Source: CAD feature listing. Evaluate the final solid. Frame: model axes, mm. Face numbers are marked on the shaded views. A direction names the side the tool comes from. Coordinates: 2 decimals unless noted, no trailing zeros. Loops run counter-clockwise (first coordinate to the right, second up) from the corner with the lowest first, then second, coordinate; pieces in that order, holes last. Notation, with made-up numbers: (69, 56.25) - (80, 56.25) arc R18 ccw to (80, 89.25) - close; hole circle Ø5 at (-32, 27.5). An arc over 180 degrees is marked (long way). Write item = value, one per line. Start each with the question number.
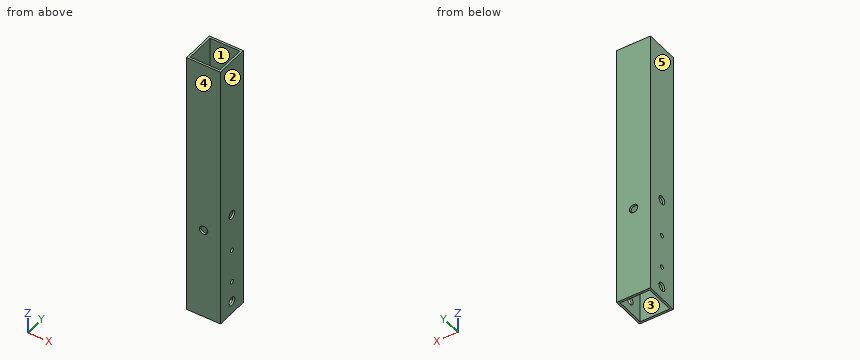
Autodesk Inventor part; units mm, degrees
ref_plane "YZ Plane" through (0, 0, 0) normal (1, 0, 0) x (0, 1, 0)
ref_plane "XZ Plane" through (0, 0, 0) normal (0, 1, 0) x (-1, 0, 0)
ref_plane "XY Plane" through (0, 0, 0) normal (0, 0, 1) x (1, 0, 0)
sketch "Sketch1" plane through (0, 0, 0) normal (0, 0, 1) x (1, 0, 0)
  line L0 (0, 0) -> (-11.1125, 0) construction
  line L1 (0, 0) -> (0, 11.1125) construction
  line L2 (-11.1125, 11.1125) -> (11.1125, 11.1125)
  line L3 (11.1125, 11.1125) -> (11.1125, -11.1125)
  line L4 (11.1125, -11.1125) -> (-11.1125, -11.1125)
  line L5 (-11.1125, -11.1125) -> (-11.1125, 11.1125)
  line L6 (-12.7, 12.7) -> (12.7, 12.7)
  line L7 (12.7, 12.7) -> (12.7, -12.7)
  line L8 (12.7, -12.7) -> (-12.7, -12.7)
  line L9 (-12.7, -12.7) -> (-12.7, 12.7)
  line L10 (-11.1125, 0) -> (-12.7, 0) construction
  line L11 (0, 11.1125) -> (0, 12.7) construction
  dimension "d0" = 25.4
  dimension "d1" = 1.5875
extrude "Extrusion1" add sketch "Sketch1" along normal blind 203.2
sketch "Sketch2" plane through (-12.7, 12.7, 0) normal (0, 1, 0) x (1, 0, 0)
  line L0 (12.7, 0) -> (12.7, -203.2) construction
  line L1 (25.4, 0) -> (25.4, -203.2) construction
  circle A0 centre (12.7, -69.85) radius 3.175
  dimension "d4" = 6.35
  dimension "d5" = 69.85
extrude "Extrusion2" cut sketch "Sketch2" against normal through all
sketch "Sketch3" plane through (12.7, -12.7, 0) normal (1, 0, 0) x (0, 0, -1)
  line L0 (0, 12.7) -> (-203.2, 12.7) construction
  line L1 (0, 23.8125) -> (-203.2, 23.8125) construction
  circle A0 centre (-79.375, 12.7) radius 3.175
  circle A1 centre (-9.525, 12.7) radius 3.175
  line L2 (0, 25.4) -> (0, 0)
  line L3 (-38.1, 23.8125) -> (-38.1, 12.7) construction
  circle A2 centre (-50.8, 12.7) radius 1.5875
  circle A3 centre (-25.4, 12.7) radius 1.5875
  dimension "d8" = 6.35
  dimension "d9" = 79.375
  dimension "d12" = 6.35
  dimension "d13" = 9.525
  dimension "d22" = 3.175
  dimension "d23" = 25.4
  dimension "d24" = 38.1
extrude "Extrusion3" cut sketch "Sketch3" against normal through all
properties part number "Upright" material "Aluminum 6061"
Item 1: Cut plane C-C (y = 8.5). Return the cut outline in (x, z), then the cut area to 3 significant figures.
Item 2: Reachability of the marked faces 1 and 2 from +Z, -Z, +X, -X, +Y, -Y: full face, straight path, thin tool, end or side. Return the list, or none.
Item 3: Cut plane A-A (x = 0). Return the cut outline in (y, z) (1 decimal).
Item 4: Cut plane B-B (z = 111). Return the cut outline in (x, y).
Item 5: Draft query along X for the marked faces 3, 4 and 5. Return one class per face: released by +X, released by -X, zero draft, split by the parting line, or undercut.
Item 6: Material intervals for L1, parallel to X at y = 11.55, z = 69.85 (3 decimals); L2, parallel to X at y = -4, z = 95, sorted ascending. Write a range as [from, to].
Responses:
q1.outline = (-12.7, 0) - (-11.11, 0) - (-11.11, 203.2) - (-12.7, 203.2) - close; (11.11, 0) - (12.7, 0) - (12.7, 203.2) - (11.11, 203.2) - close
q1.area = 645 mm2
q2.face_1 = +Z, -Z
q2.face_2 = +Z, -Z, +X, +Y, -Y
q3.outline = (-12.7, 0) - (-11.1, 0) - (-11.1, 66.7) - (-12.7, 66.7) - close; (-12.7, 73) - (-11.1, 73) - (-11.1, 203.2) - (-12.7, 203.2) - close; (11.1, 0) - (12.7, 0) - (12.7, 66.7) - (11.1, 66.7) - close; (11.1, 73) - (12.7, 73) - (12.7, 203.2) - (11.1, 203.2) - close
q4.outline = (-12.7, -12.7) - (12.7, -12.7) - (12.7, 12.7) - (-12.7, 12.7) - close; hole (-11.11, -11.11) - (11.11, -11.11) - (11.11, 11.11) - (-11.11, 11.11) - close
q5.face_3 = undercut
q5.face_4 = zero draft
q5.face_5 = released by -X
q6.L1 = [-12.7, -3.175], [3.175, 12.7]
q6.L2 = [-12.7, -11.11], [11.11, 12.7]
